```python
from build123d import *

# Parameters (mm, degrees)
F0_R     = 15.875
F0_R_2   = 14.2875
F1_DEPTH = 101.6
F3_R     = 6.35
F4_DEPTH = 25.4
F6_R     = 6.35
F7_DEPTH = 25.4


with BuildPart() as f1:
    # F0 (on Front) → F1 (new body)
    with BuildSketch(Plane.XZ):
        Circle(F0_R)
        Circle(F0_R_2, mode=Mode.SUBTRACT)
    extrude(amount=F1_DEPTH)

    # F3 (on offset) → F4 (cut)
    with BuildSketch(Plane.XY.offset(28.575)):
        with Locations((0, -33.02)):
            Circle(F3_R)
    extrude(amount=-F4_DEPTH, mode=Mode.SUBTRACT)

    # F6 (on offset) → F7 (cut)
    with BuildSketch(Plane.XY.offset(-28.575)):
        with Locations((0, -9.525)):
            Circle(F6_R)
    extrude(amount=F7_DEPTH, mode=Mode.SUBTRACT)


solid = f1.part
```
Geometry check sheet. Reference: the model listing, model coordinates, mm. A direction names the side the tool comes from. Round coordinates to 2 decimals unless told otherwise and drop trailing zeros. Loops run counter-clockwise (first coordinate to the right, second up) from the corner with the lowest first, then second, coordinate; pieces in that order, holes last. Notation, with made-up numbers: M 52,-39.5 L 109,-39.5 A21 ccw 109,-25.5 Z; hole C -7,41.25 d3. An arc over 180 degrees is marked long. Return JSON: item names as keys, results as strings. Group by question number.
(1) Set-up check for faces 1 (the face through (2.93, -38.654, 14.362)), 2 (the face through (7.33, -50.09, -14.08)): record each of +Z, -Z, +X, -X, +Y, -Y from which the full face is reachable in a straight line by a thin tool's end or side.
(2) Scan lines: line 1 along Y through (x, z) = (0, 14.55); line 2 along Y through (x, z) = (0, -15) (3 decimals); line 3 along Z through (x, y) = (-11.5, -89). Record each from-to range of solid material in increasing order. Write a range as [from, to].
(3) Mould release check, pull along Y, two halves, no side actions. Record for faces 3 (the face through (-11.83, 0, 8.31)), 4 (the face through (-11.83, -101.6, 8.31)), 5 (the face through (3.41, -4.17, -14.36)): pulls with the +Y half, pulls with the -Y half, needs draft (parallel to the pull), parting line crosses it, or undercut.
(4) Go/stop test with flat-tipped pins: pin 1 (10 mm diameter, centred on y = -71, z = 4, fed in from -X) (3 decimals); pin 2 (12 mm diameter, centred on y = -38, z = 8, fed in from -X); pin 3 (1 mm diameter, centred on y = -39.5, z = -10.5, fed in from +X); pin 4 (10 mm diameter, centred on y = -48.5, z = -6, fed in from +X). Record where each tip stops, or that it passes through.
(5) Section check C-C, the plane x = -11. Enter the section's corners in (y, z), and give its area (3 significant figures).
(6) Section check B-B, the plane z = 0. Enter the section's corners in (x, y) (1 decimal).
(7) Section check A-A, the plane x = 0. Enter the section's corners in (y, z) (1 decimal), and give its area (3 significant figures).
Data:
{
 "1": {"face 1": "+Z", "face 2": "+Y, -Y"},
 "2": {"line 1": "[-101.6, -39.37], [-26.67, 0]", "line 2": "[-101.6, -15.875], [-3.175, 0]", "line 3": "[-10.94, -8.48], [8.48, 10.94]"},
 "3": {"face 3": "pulls with the +Y half", "face 4": "pulls with the -Y half", "face 5": "undercut"},
 "4": {"pin 1": "x = -15.875", "pin 2": "x = -15.75", "pin 3": "x = 12.33", "pin 4": "x = 15.84"},
 "5": {"outline": "M -101.6,-11.45 L 0,-11.45 L 0,-9.12 L -101.6,-9.12 Z; M -101.6,9.12 L 0,9.12 L 0,11.45 L -101.6,11.45 Z", "area": "473 mm²"},
 "6": {"outline": "M -15.9,-101.6 L -14.3,-101.6 L -14.3,0 L -15.9,0 Z; M 14.3,-101.6 L 15.9,-101.6 L 15.9,0 L 14.3,0 Z"},
 "7": {"outline": "M -101.6,-15.9 L -15.9,-15.9 L -15.9,-14.3 L -101.6,-14.3 Z; M -101.6,14.3 L -39.4,14.3 L -39.4,15.9 L -101.6,15.9 Z; M -26.7,14.3 L 0,14.3 L 0,15.9 L -26.7,15.9 Z; M -3.2,-15.9 L 0,-15.9 L 0,-14.3 L -3.2,-14.3 Z", "area": "282 mm²"}
}
